Model file for the job. Use its own axes, mm. Give positions to 0.01 mm unless a question says otherwise; leave off trailing zeros. One line per item, written item: value. Start each with the question number.
(1) Mould opens along Z. For faces 1 (the face through (-2.32, -0.52, -2.8)), 2 (the face through (0.864, 2.744, -2.789)) say: pulls with the +Z half, pulls with the -Z half, needs draft (parallel to the pull), parting line crosses it, or undercut.
(2) Probe L1, parallel to Z at x = -0.75, y = 58; L2, parallel to Y at x = 1.75, z = -17.5; L3, parallel to Y at x = -0.5, z = -37.5. List the from-to ranges inside material, lowest first.
(3) Drop flat-ended pins along their axis: P1, Ø1, axis at x = 0.5, z = -37, coming from the -Y side; P2, Ø5, axis at y = 12.5, z = -22.5, coming from the +X side; P3, Ø1, axis at x = 0, y = 59, coming from the -Z side. Give the stop position or say it passes through.
Autodesk Inventor part; units mm, degrees
ref_plane "Arbeitsebene1" through (0, 0, -5.5) normal (0, 0, 1) x (1, 0, 0)
ref_plane "Arbeitsebene2" through (0, 0, -5.5) normal (0, 0, -1) x (-1, 0, 0)
ref_plane "YZ Plane" through (0, 0, 0) normal (1, 0, 0) x (0, 1, 0)
sketch "Skizze1" plane through (0, 0, 0) normal (0, 0, 1) x (0, 1, 0)
  circle A0 centre (0, 0) radius 2.75
  dimension "d0" = 5.5
sketch "Skizze2" plane through (0, 0, 0) normal (1, 0, 0) x (0, 1, 0)
  arc A0 (0, -5.5) -> (63.45, -42.1329) centre (42.3, -5.5) ccw
  line L0 (63.45, -42.1329) -> (67.5203, -39.7829)
  line L1 (42.3, -5.5) -> (42.3, -47.8) construction
  point P0 (0, 0)
  point P1 (0, 0)
  dimension "d3" = 5.5
  dimension "d4" = 42.3
  dimension "d5" = 4.7
  dimension "d27" = 60
ref_plane "Arbeitsebene1" through (0, 0, -5.5) normal (0, 0, 1) x (1, 0, 0)
sketch "Skizze3" plane through (0, 0, -5.5) normal (0, 0, 1) x (1, 0, 0)
  circle A0 centre (0, 0) radius 3
  dimension "d11" = 6
ref_plane "Arbeitsebene2" through (0, 0, -5.5) normal (0, 0, -1) x (-1, 0, 0)
sketch "Skizze4" plane through (0, 0, -5.5) normal (0, 0, -1) x (-1, 0, 0)
  circle A0 centre (0, 0) radius 3
loft "Erhebung2" add profiles "Skizze1", "Skizze3"
sweep "Sweeping3" add profiles "Skizze4" path "Skizze2"
shell "Wandung2" thickness 0.5 removed faces 2 at (-0.6079, 0.6861, 0) at (-0.7485, 67.8519, -40.3572)
properties part number "Tube" material "Kupfer"
Answers follow:
1. face 1: undercut
1. face 2: pulls with the +Z half
2. L1: z = -47.89 to -47.34, -42.2 to -41.63
2. L2: y = -0.8 to -0.12, 3.6 to 4.29
2. L3: y = 10.3 to 11.02, 18.55 to 19.41, 65.56 to 66.2
3. P1: stops at y = 9.31
3. P2: passes through
3. P3: stops at z = -47.8
